Source: CAD feature listing. Evaluate the final solid. Frame: model axes, mm. A direction names the side the tool comes from. Give positions to 0.01 mm unless a question says otherwise; leave off trailing zeros. Order: outer loops, then holes, each group sorted by start corner. A loop starts at its lowest first (then second) coordinate and runs counter-clockwise, first axis right, second up. Notation, with made-up numbers: M -0.5,57 L 48.5,57 A32 ccw 48.5,93 Z; hole C 59,21 d1. An arc over 180 degrees is marked long. Use CSV: the item, a comma, the result in double quotes. Start each with the question number.
1. Section query A-A, the plane x = 18.5. Return the cut outline in (y, z).
2. Section query D-D, the plane x = -16. Return the cut outline in (y, z), plus the area to 3 significant figures.
3. Pin query (flat end, axial travel): P1, Ø3, axis at y = 10, z = 6, coming from the +X side; P2, Ø20, axis at x = -8.5, y = -2, coming from the +Z side; P3, Ø2, axis at x = 10, z = 20.5, coming from the -Y side; P4, Ø0.6, axis at x = 12.5, z = 23, coming from the -Y side. Return the tip coordinate at first contact, or that it passes through.
4. Reachability of faces 1 (the flat face through (-4.5, 15, 17)), 2 (the cylindrical face through (-19.79, -17.32, 1.97)) from +Z, -Z, +X, -X, +Y, -Y: full face, straight path, thin tool, end or side. Return the list, or none.
5. Mould query, pull axis X, two halves, no side actions, for faces 3 (the flat face through (-1.5, 15, 17)), 4 (the flat face through (17, 11.885, 17)). Classes: released by +X, released by -X, zero draft, split by the parting line, or undercut.
6. Section query C-C, the plane z = 3. Return the cut outline in (x, y), plus the area to 3 significant figures.
7. Section query B-B, the plane y = -18.5. Return the cut outline in (x, z).
8. Line query: line 1 along Y through (x, z) = (-18.5, 2.3); line 2 along Y through (x, z) = (-18.5, 22.5); line 3 along Y through (x, z) = (0, 18.25). Output: solid intervals per line, ascending. Write a range as [from, to].
from build123d import *

# Parameters (mm, degrees)
SKETCH_1_W          = 43
SKETCH_1_H          = 43
SKETCH_1_R          = 1.75
EXTRUDE_1_DEPTH     = 30
SKETCH_2_W          = 43
SKETCH_2_H          = 33.384643537
SKETCH_2_R          = 1.75
CUT_EXTRUDE_1_DEPTH = 26
SKETCH_3_W          = 2
SKETCH_3_H          = 6.115356463
CUT_EXTRUDE_2_DEPTH = 26


with BuildPart() as part:
    # 草图1 → 凸台-拉伸1 (new body)
    with BuildSketch(Plane.XY):
        Rectangle(SKETCH_1_W, SKETCH_1_H)
        with Locations((-18.5, 18.5)):
            Circle(SKETCH_1_R, mode=Mode.SUBTRACT)
        with Locations((-18.5, -18.5)):
            Circle(SKETCH_1_R, mode=Mode.SUBTRACT)
        with Locations((18.5, -18.5)):
            Circle(SKETCH_1_R, mode=Mode.SUBTRACT)
        with Locations((18.5, 18.5)):
            Circle(SKETCH_1_R, mode=Mode.SUBTRACT)
    extrude(amount=EXTRUDE_1_DEPTH)

    # 草图2 → 切除-拉伸1 (cut)
    with BuildSketch(Plane.XY.offset(30)):
        with Locations((0, -4.807678231)):
            Rectangle(SKETCH_2_W, SKETCH_2_H)
        with Locations((-18.5, -18.5)):
            Circle(SKETCH_2_R, mode=Mode.SUBTRACT)
        with Locations((18.5, -18.5)):
            Circle(SKETCH_2_R, mode=Mode.SUBTRACT)
    extrude(amount=-CUT_EXTRUDE_1_DEPTH, mode=Mode.SUBTRACT)

    # 草图3 → 切除-拉伸2 (cut)
    with BuildSketch(Plane.XY.offset(30)):
        with Locations((-11.5, 14.942321769)):
            Rectangle(SKETCH_3_W, SKETCH_3_H)
        with Locations((-8.5, 14.942321769)):
            Rectangle(SKETCH_3_W, SKETCH_3_H)
        with Locations((-5.5, 14.942321769)):
            Rectangle(SKETCH_3_W, SKETCH_3_H)
        with Locations((-2.5, 14.942321769)):
            Rectangle(SKETCH_3_W, SKETCH_3_H)
        with Locations((0.5, 14.942321769)):
            Rectangle(SKETCH_3_W, SKETCH_3_H)
        with Locations((3.5, 14.942321769)):
            Rectangle(SKETCH_3_W, SKETCH_3_H)
        with Locations((6.5, 14.942321769)):
            Rectangle(SKETCH_3_W, SKETCH_3_H)
        with Locations((9.5, 14.942321769)):
            Rectangle(SKETCH_3_W, SKETCH_3_H)
        with Locations((12.5, 14.942321769)):
            Rectangle(SKETCH_3_W, SKETCH_3_H)
    extrude(amount=-CUT_EXTRUDE_2_DEPTH, mode=Mode.SUBTRACT)


solid = part.part
Result set:
1,outline,"M -21.5,0 L -20.25,0 L -20.25,4 L -21.5,4 Z; M -16.75,0 L 16.75,0 L 16.75,30 L 11.88,30 L 11.88,4 L -16.75,4 Z; M 20.25,0 L 21.5,0 L 21.5,30 L 20.25,30 Z"
2,outline,"M -21.5,0 L 21.5,0 L 21.5,30 L 11.88,30 L 11.88,4 L -21.5,4 Z"
2,area,"422 mm2"
3,P1,"through"
3,P2,"z = 4"
3,P3,"y = 11.88"
3,P4,"y = 18"
4,face 1,"+Z, -Y"
4,face 2,"+Z, -Z"
5,face 3,"undercut"
5,face 4,"zero draft"
6,outline,"M -21.5,-21.5 L 21.5,-21.5 L 21.5,21.5 L -21.5,21.5 Z; hole C -18.5,-18.5 d3.5; hole C -18.5,18.5 d3.5; hole C 18.5,-18.5 d3.5; hole C 18.5,18.5 d3.5"
6,area,"1,810 mm2"
7,outline,"M -21.5,0 L -20.25,0 L -20.25,4 L -21.5,4 Z; M -16.75,0 L 16.75,0 L 16.75,4 L -16.75,4 Z; M 20.25,0 L 21.5,0 L 21.5,4 L 20.25,4 Z"
8,line 1,"[-21.5, -20.25], [-16.75, 16.75], [20.25, 21.5]"
8,line 2,"[11.88, 16.75], [20.25, 21.5]"
8,line 3,"[18, 21.5]"
